```python
from build123d import *

# Parameters (mm, degrees)
SKETCH3_R          = 63.5
SKETCH3_R_2        = 51.1302
SKETCH5_R          = 63.5
SKETCH5_R_2        = 42.73738
CUT_EXTRUDE1_DEPTH = 25.4


with BuildPart() as part:
    # Sketch1 → Revolve1 (revolve)
    with BuildSketch(Plane.XY, mode=Mode.PRIVATE) as revolve1_sk:
        Polygon((-110.49, -63.5), (-58.928, -63.5), (-58.928, -57.0357), (-110.49, -57.3786), align=None)
    revolve(revolve1_sk.sketch.rotate(Axis((-110.49, 0, 0), (1, 0, 0)), 270), axis=Axis((-110.49, 0, 0), (1, 0, 0)))


with BuildPart() as body_2:
    # Sketch2 → Revolve2 (revolve)
    with BuildSketch(Plane.XY, mode=Mode.PRIVATE) as revolve2_sk:
        Polygon((57.3786, 110.49), (57.0357, 58.928), (63.5, 58.928), (63.5, 110.49), align=None)
    revolve(revolve2_sk.sketch.rotate(Axis((0, 0, 0), (0, 1, 0)), 90), axis=Axis((0, 0, 0), (0, 1, 0)))


with BuildPart() as sweep1_tool:
    # Sweep1: sweep along a path in Sketch4
    with BuildLine(Plane.XY) as sweep1_path:
        ThreePointArc((-58.928, 0), (-17.259612, 17.259612), (0, 58.928))
    # Sketch3 → Sweep1 (sweep)
    with BuildSketch(Plane(origin=(-58.928, 0, 0), x_dir=(0, 0, -1), z_dir=(1, 0, 0))):
        Circle(SKETCH3_R)
        Circle(SKETCH3_R_2, mode=Mode.SUBTRACT)
    sweep(path=sweep1_path.line)


with BuildPart() as part_1:
    add(part.part)


with BuildPart() as part_2:
    # Sweep1: joined with sweep1_tool
    add(part_1.part.fuse(sweep1_tool.part, body_2.part, tol=0.00001))

    # Sketch5 → Cut-Extrude1 (cut)
    with BuildSketch(Plane(origin=(0, 110.49, 0), x_dir=(1, 0, 0), z_dir=(0, 1, 0))):
        with Locations(Location((0, 0, 0), (0, 0, 158.125167))):
            Circle(SKETCH5_R)
        Circle(SKETCH5_R_2, mode=Mode.SUBTRACT)
    extrude(amount=-CUT_EXTRUDE1_DEPTH, mode=Mode.SUBTRACT)


solid = part_2.part
```
Check sheet for the modelled part. Datum: model origin and axes. Units: mm. A direction names the side the tool comes from. Round coordinates to 2 decimals unless told otherwise and drop trailing zeros. Loops run counter-clockwise (first coordinate to the right, second up) from the corner with the lowest first, then second, coordinate; pieces in that order, holes last. Notation, with made-up numbers: (1.25, -28.5) - (39.25, -28.5) arc R15 ccw to (39.25, -14.5) - close; hole circle Ø4 at (80.25, -34.75). An arc over 180 degrees is marked (long way). Answer as a JSON object with one key per item and string values. Group by question number.
Q1. Set-up check for faces 4 (the face through (49, 85.09, 30)), 5 (the face through (-85.07, -2.515, -57.154)), 6 (the face through (-21, 58.928, -47)): record each of +Z, -Z, +X, -X, +Y, -Y from which the full face is reachable in a straight line by a thin tool's end or side.
Q2. Mould release check, pull along Z, two halves, no side actions. Record for faces 1 (the face through (-84.35, -53.54, 34.14)), 2 (the face through (-17.158, 71.826, -54.484)), 3 (the face through (-110.49, 56, 14)): released by +Z, released by -Z, zero draft, split by the parting line, or undercut.
Q3. Gauge pin test, flat ends, axial feed: P1, Ø12, axis at x = -15, y = -48.5, coming from the -Z side; P2, Ø3, axis at x = -74, y = 9.5, coming from the +Z side; P3, Ø1.5, axis at x = 31.5, y = 67, coming from the -Z side; P4, Ø4, axis at x = -74, y = -0.5, coming from the -Z side. Record the tip position at first contact, or that the pin passes through.
Q4. Scan lines: line 1 along Z through (x, y) = (-23.5, 14); line 2 along Y through (x, z) = (-79, -31); line 3 along Y through (x, z) = (-70, -17). Record each from-to range of solid material in increasing order. Write a range as [from, to].
Q5. Sectioned sample at A-A, the plane x = -74. Enter the section's corners in (y, z), plus the area to 3 significant figures.
Solution:
{
 "1": {"face 4": "+Z, -Z, +X, -X, +Y", "face 5": "-X", "face 6": "+Y"},
 "2": {"face 1": "split by the parting line", "face 2": "undercut", "face 3": "zero draft"},
 "3": {"P1": "stops at z = -37.65", "P2": "stops at z = 62.99", "P3": "stops at z = -55.56", "P4": "stops at z = -63.5"},
 "4": {"line 1": "z = [-63.48, -51.1], [51.1, 63.48]", "line 2": "y = [-55.42, -48.03], [48.03, 55.42]", "line 3": "y = [-61.18, -54.52], [54.52, 61.18]"},
 "5": {"outline": "circle Ø127 at (0, 0); hole circle Ø114.27 at (0, 0)", "area": "2,410 mm²"}
}
